from build123d import *

# Parameters (mm, degrees)
EXTRUDE_1_DEPTH      = 2
SKETCH_2_R           = 3
EXTRUDE_2_DEPTH      = 8
SKETCH_3_R           = 3
EXTRUDE_3_DEPTH      = 4
EXTRUDE_3_DEPTH_BACK = 6
EXTRUDE_4_DEPTH      = 2
SCALE_3_SCALE        = 3.5


with BuildPart() as part:
    # 草图1 → 凸台-拉伸1 (new body)
    with BuildSketch(Plane.XY):
        with BuildLine():
            Line((-4.5, -20), (-4.5, 20))
            ThreePointArc((-4.5, 20), (0, 24.5), (4.5, 20))
            Line((4.5, 20), (4.5, -20))
            ThreePointArc((4.5, -20), (0, -24.5), (-4.5, -20))
        make_face()
    extrude(amount=EXTRUDE_1_DEPTH)

    # 草图2 → 凸台-拉伸2 (add)
    with BuildSketch(Plane.XY.offset(2)):
        Circle(SKETCH_2_R)
    extrude(amount=EXTRUDE_2_DEPTH)

    # 草图3 → 凸台-拉伸3 (add, two sides)
    with BuildSketch(Plane.XY.offset(2)) as extrude_3_sk:
        with Locations((0, -20.775035614)):
            Circle(SKETCH_3_R)
    extrude(amount=EXTRUDE_3_DEPTH)
    extrude(extrude_3_sk.sketch, amount=-EXTRUDE_3_DEPTH_BACK)

    # 草图4 → 凸台-拉伸4 (add)
    with BuildSketch(Plane.XY.offset(2)):
        Polygon((-4.5, 60), (-4.5, 20), (4.5, 20), (4.5, 56.272077939), (30.148232278, 81.920310217), (23.784271247, 88.284271247), align=None)
    extrude(amount=-EXTRUDE_4_DEPTH)


with BuildPart() as part_1:
    # 缩放比例3: scaled about (3.511892573, 26.803081313, 1.433505164)
    add(part.part.scale(SCALE_3_SCALE).moved(Location((-8.779731433, -67.007703283, -3.58376291))))


solid = part_1.part
Can you work these out from the model? Positions are in its coordinate system, mm. A direction names the side the tool comes from. Coordinates: 2 decimals unless noted, no trailing zeros. Loops run counter-clockwise (first coordinate to the right, second up) from the corner with the lowest first, then second, coordinate; pieces in that order, holes last. Notation, with made-up numbers: (81.25, 13.25) - (123.25, 13.25) arc R32 cw to (123.25, 45.25) - close; hole circle Ø1 at (-22, 17.25). An arc over 180 degrees is marked (long way). Answer as a JSON object with one key per item and string values. Group by question number.
Item 1: If we section it at D-D (z = 26): List the corners of the cut face in (x, y) for me.
Item 2: For pin 1 (10.5 mm diameter, centred on x = -5.5, y = -137.5, fed in from +Z); pin 2 (5.5 mm diameter, centred on y = -13.5, z = 0, fed in from +X); pin 3 (1.5 mm diameter, centred on x = 37, z = -4, fed in from +Y); pin 4 (10 mm diameter, centred on x = 14.5, y = -2.5, fed in from +Z), each with a flat end and sliding along its axis, tell me the tip position at first contact or that it passes through.
Item 3: On a 3-axis mill with a long thin cutter (end or side, diameter ignored), from which of +Z, -Z, +X, -X, +Y, -Y can I reach the whole of each face in a straight line? I mean faces 4 (the face through (-9, -140, -17.584)), 5 (the face through (6.97, -5, 0)), 6 (the face through (-3.935, -149.036, -10.486)), 7 (the face through (25.66, 193.18, -0.03)), 8 (the face through (-3.935, -149.036, 10.318)). Say none if no direction works.
Item 4: If we section it at B-B (y = 8.5): List the corners of the cut face in (x, z) for me.
Item 5: If we section it at A-A (z = 0): List the corners of the cut face in (x, y) for me, plus the area to 3 significant figures.
Item 6: If we mould it in two halves opening along Y, with no side actions, what happens to faces 1 (the face through (85.76, 230.69, -0.03)), 2 (the face through (-11.056, -77.258, 17.22)), 3 (the face through (-9, -140, 17.416))? For each: released by +Y, released by -Y, zero draft, split by the parting line, or undercut.
Item 7: If we section it at C-C (x = 84.5): List the corners of the cut face in (y, z) for me, plus the area to 3 significant figures.
Item 8: If I drill on L1, parallel to Z at x = -14, y = 31.5; L2, parallel to X at y = -36.5, z = 0; L3, parallel to Y at x = -1.5, z = 19.5, over which ranges is the centre line in solid material (lowest first)? Write a range as from..to.
Returned:
{
 "1": {"outline": "circle Ø21 at (-8.78, -67.01)"},
 "2": {"pin 1": "stops at z = 17.42", "pin 2": "stops at x = 6.97", "pin 3": "stops at y = 205.15", "pin 4": "passes through"},
 "3": {"face 4": "-Z, +X, -X, +Y, -Y", "face 5": "+Z, -Z, +X, -Y", "face 6": "-Z", "face 7": "+Z, -Z, -X, +Y", "face 8": "+Z"},
 "4": {"outline": "(-24.53, -3.58) - (6.97, -3.58) - (6.97, 3.42) - (-24.53, 3.42) - close"},
 "5": {"outline": "(-24.53, -137.01) arc R15.75 ccw to (6.97, -137.01) - (6.97, 129.94) - (96.74, 219.71) - (74.47, 241.99) - (-24.53, 142.99) - close", "area": "13,200 mm²"},
 "6": {"face 1": "released by +Y", "face 2": "undercut", "face 3": "zero draft"},
 "7": {"outline": "(207.47, -3.58) - (231.95, -3.58) - (231.95, 3.42) - (207.47, 3.42) - close", "area": "171 mm²"},
 "8": {"L1": "z = -3.58..3.42", "L2": "x = -24.53..6.97", "L3": "y = -74.57..-59.44"}
}
